Solid Edge part; units mm, degrees
sketch "Sketch1" plane through (0, 0, 0) normal (0, 0, 1) x (1, 0, 0)
  circle A0 centre (0, 0) radius 10
extrude "Protrusion1" add sketch "Sketch1" along normal blind 5.5
sketch "Sketch2" plane through (0, 0, 0) normal (0, 0, -1) x (1, 0, 0)
  circle A0 centre (0, 0) radius 5
extrude "Protrusion2" add sketch "Sketch2" along normal blind 74.5
sketch "Sketch3" plane through (0, 0, -74.5) normal (0, 0, -1) x (1, 0, 0)
  circle A0 centre (0, 0) radius 4.9997
extrude "Cutout1" cut sketch "Sketch3" against normal blind 26 flip side to cut
chamfer "Chamfer_1" distance 0.75 angle 45 1 edges at (-4.9997, 0, -74.5)
sketch "Sketch4" plane through (0, 0, 5.5) normal (0, 0, 1) x (1, 0, 0)
  line L0 (-1.7321, 3) -> (1.7321, 3)
  line L1 (3.4641, 0) -> (1.7321, 3)
  line L2 (1.7321, -3) -> (3.4641, 0)
  line L3 (-1.7321, -3) -> (1.7321, -3)
  line L4 (-3.4641, 0) -> (-1.7321, -3)
  line L5 (-1.7321, 3) -> (-3.4641, 0)
extrude "Cutout2" cut sketch "Sketch4" against normal blind 3.6667
sketch "Sketch5" plane through (0, 0, 0) normal (0, -1, 0) x (1, 0, 0)
  line L0 (10, 5.5) -> (4.5, 0)
  line L1 (4.5, 0) -> (10, 0)
  line L2 (10, 0) -> (10, 5.5)
revolve "RevolvedCutout1" cut sketch "Sketch5" angle 360 about axis through (0, 0, 14.0017) along (0, 0, -1)
properties part number "300546"
Part model, mm, in its own coordinate system. A direction names the side the tool comes from. Round coordinates to 2 decimals unless told otherwise and drop trailing zeros. Write each loop counter-clockwise with the first axis right and the second up, starting at its lowest first coordinate (ties: lowest second). Pieces come first, ordered by that corner, then holes. Notation, with made-up numbers: M -35.5,86.25 L -18.5,86.25 A31 cw -18.5,124.25 Z; hole C 18.25,79.5 d9. An arc over 180 degrees is marked long. Return JSON: item names as keys, results as strings. Group by question number.
(1) Saw through at B-B on z = 1. Write the cut outline in (x, y), then the cut area to 3 significant figures.
(2) Which spindle directions (+Z, -Z, +X, -X, +Y, -Y) get a long thin tool onto all of the face, cutting with end or side? Do faces 1 (the face through (-2.6, -1.5, 3.7)), 2 (the face through (-1.08, -4.88, -23.91)), 3 (the face through (-2.4, 2.4, 5.5)). Say none if no direction does.
(3) Drill centre lines: probe 1 along X at (y, z) = (4, -34.5); probe 2 along Z at (x, y) = (1, 6.25); probe 3 along Z at (x, y) = (-2.25, -0.5). Where is each one in solid material? Low to high.
(4) Pin check, flat tips, straight feed: pin 1 Ø1.5 at (x, y) = (7, 0) entering from -Z; pin 2 Ø4 at (x, z) = (0, -27) entering from +Y; pin 3 Ø1.7 at (x, z) = (-0.5, 3.5) entering from +Y. Stop position of each tip, or through.
(5) Two-plate mould, pull along X, no slides. Class faces 4 (the face through (0, -3, 4)), 5 (the face through (4.77, -1.5, -61.3)), 6 (the face through (0, 0, -74.5)): +X half, -X half, draft (parallel to the pull), parting line (faces both ways), or undercut.
(6) Saw through at C-C on z = -51.5. Write the cut outline in (x, y).
Returned:
{
 "1": {"outline": "C 0,0 d11", "area": "95.0 mm²"},
 "2": {"face 1": "+Z", "face 2": "-Z", "face 3": "+Z, +X, -X, +Y, -Y"},
 "3": {"probe 1": "-3 to 3", "probe 2": "1.83 to 5.5", "probe 3": "-74.5 to 1.83"},
 "4": {"pin 1": "z = 1.75", "pin 2": "y = 5", "pin 3": "y = 8.84"},
 "5": {"face 4": "undercut", "face 5": "parting line", "face 6": "draft"},
 "6": {"outline": "C 0,0 d10"}
}
